Input: part model. Units: mm. Frame: model coordinates. A direction names the side the tool comes from. Round coordinates to 2 decimals unless told otherwise and drop trailing zeros. Loops run counter-clockwise (first coordinate to the right, second up) from the corner with the lowest first, then second, coordinate; pieces in that order, holes last.
(1) Cut plane D-D, the plane y = -6. Give the number of separate pieces and of enclosed holes in the cut face, and give its area (3 significant figures).
(2) Cut plane A-A, the plane z = -5. Output: boundary loops of the cut face in (x, y), and give its area (3 significant figures).
(3) Line query: line 1 (Y direction, x = 0, z = 14.7); line 2 (X direction, y = -4.5, z = 9); line 3 (Y direction, x = 6, z = 7.25). Output: solid intervals per line, ascending.
(4) Draft query along X for faces 1 (the face through (-0.22, 11.21, 13.82)), 2 (the face through (4.737, 0.052, -3.402)), 3 (the face through (0, -2, -6.9)), 4 (the face through (-1.5, -0.07, 1.63)). Return one class per face: released by +X, released by -X, zero draft, split by the parting line, or undercut.
(5) Cut plane C-C, the plane y = 0. Output: boundary loops of the cut face in (x, z).
(6) Access query for faces 5 (the face through (6.466, -2.681, 14.514)), 6 (the face through (-11.747, -4.917, 4.93)), 7 (the face through (3, 3.35, -3)), 8 (the face through (-4.737, -0.052, -3.402)). Directions: +Z, -Z, +X, -X, +Y, -Y. A direction counts if a zero-diameter tool reaches every point of the face in a straight line with its end or side. Return the directions, or none.
(7) First-contact query: pin 1 Ø4 at (x, y) = (8.25, -4.76) entering from +Z; pin 2 Ø8 at (x, z) = (10, 9.5) entering from +Y; pin 3 Ø5 at (x, y) = (0, 0) entering from +Z; pin 4 Ø10 at (x, z) = (-11.5, 12) entering from -Y. Flat tips, straight axial feed; report the tip coordinate or a pass-through.
from build123d import *

# Parameters (mm, degrees)
SKETCH_R        = 15
SKETCH_R_2      = 1.7
PAD_DEPTH       = 16
PAD001_DEPTH    = 6.9
SKETCH006_R     = 3.5
POCKET003_DEPTH = 6.9
SKETCH003_R     = 1.5
POCKET004_DEPTH = 17.3
SKETCH008_R     = 7
POCKET_DEPTH    = 2.5
SKETCH009_R     = 3.5
POCKET005_DEPTH = 10
CHAMFER_SIZE    = 1.5
CHAMFER001_SIZE = 1.7
CHAMFER002_SIZE = 1.7
CHAMFER003_SIZE = 1.7
CHAMFER004_SIZE = 0.5


with BuildPart() as part:
    # Sketch → Pad (new body)
    with BuildSketch(Plane.XY):
        Circle(SKETCH_R)
        with Locations((0, 9.526279)):
            Circle(SKETCH_R_2, mode=Mode.SUBTRACT)
        with Locations((-8.25, -4.76314)):
            Circle(SKETCH_R_2, mode=Mode.SUBTRACT)
        with Locations((8.25, -4.76314)):
            Circle(SKETCH_R_2, mode=Mode.SUBTRACT)
    extrude(amount=PAD_DEPTH)

    # Sketch004 → Pad001 (new body)
    with BuildSketch(Plane(origin=(0, 0, 0), x_dir=(1, 0, 0), z_dir=(0, 0, -1))):
        with BuildLine():
            Line((-3.35, 3.35), (3.35, 3.35))
            ThreePointArc((3.35, -3.35), (4.737615, 0), (3.35, 3.35))
            Line((3.35, -3.35), (-3.35, -3.35))
            ThreePointArc((-3.35, 3.35), (-4.737615, 0), (-3.35, -3.35))
        make_face()
    extrude(amount=PAD001_DEPTH)

    # Sketch006 → Pocket003 (cut)
    with BuildSketch(Plane(origin=(0, 0, -6.9), x_dir=(1, 0, 0), z_dir=(0, 0, -1))):
        with Locations((0, 6)):
            Circle(SKETCH006_R)
        with Locations((0, -6)):
            Circle(SKETCH006_R)
    extrude(amount=-POCKET003_DEPTH, mode=Mode.SUBTRACT)

    # Sketch003 → Pocket004 (cut)
    with BuildSketch(Plane(origin=(0, 0, -6.9), x_dir=(1, 0, 0), z_dir=(0, 0, -1))):
        Circle(SKETCH003_R)
    extrude(amount=-POCKET004_DEPTH, mode=Mode.SUBTRACT)

    # Sketch008 → Pocket (cut)
    with BuildSketch(Plane.XY.offset(16)):
        Circle(SKETCH008_R)
    extrude(amount=-POCKET_DEPTH, mode=Mode.SUBTRACT)

    # Sketch009 → Pocket005 (cut)
    with BuildSketch(Plane(origin=(0, 0, 0), x_dir=(1, 0, 0), z_dir=(0, 0, -1))):
        with Locations((8.25, 4.76314)):
            Circle(SKETCH009_R)
        with Locations((-8.25, 4.76314)):
            Circle(SKETCH009_R)
        with Locations((0, -9.526279)):
            Circle(SKETCH009_R)
    extrude(amount=-POCKET005_DEPTH, mode=Mode.SUBTRACT)

    # Chamfer
    chamfer_edges = [part.edges().sort_by_distance(p)[0] for p in [
        (-15, 0, 0),
    ]]
    chamfer(chamfer_edges, length=CHAMFER_SIZE)

    # Chamfer001
    chamfer001_edges = [part.edges().sort_by_distance(p)[0] for p in [
        (-9.95, -4.76314, 10),
    ]]
    chamfer(chamfer001_edges, length=CHAMFER001_SIZE)

    # Chamfer002
    chamfer002_edges = [part.edges().sort_by_distance(p)[0] for p in [
        (6.55, -4.76314, 10),
    ]]
    chamfer(chamfer002_edges, length=CHAMFER002_SIZE)

    # Chamfer003
    chamfer003_edges = [part.edges().sort_by_distance(p)[0] for p in [
        (-1.7, 9.526279, 10),
    ]]
    chamfer(chamfer003_edges, length=CHAMFER003_SIZE)

    # Chamfer004
    chamfer004_edges = [part.edges().sort_by_distance(p)[0] for p in [
        (-7, 0, 16),
    ]]
    chamfer(chamfer004_edges, length=CHAMFER004_SIZE)


solid = part.part
Reported:
1. separate pieces: 3
1. enclosed holes: 0
1. area: 253 mm2
2. outline: (-3.35, -3.35) - (-2.29, -3.35) arc R3.5 cw to (2.29, -3.35) - (3.35, -3.35) arc R4.74 ccw to (3.35, 3.35) - (2.29, 3.35) arc R3.5 cw to (-2.29, 3.35) - (-3.35, 3.35) arc R4.74 ccw to start; hole circle Ø3 at (0, 0)
2. area: 45.3 mm2
3. line 1: y = -15 to -7, 7 to 7.83, 11.23 to 15
3. line 2: x = -14.31 to -11.74, -4.76 to 4.76, 11.74 to 14.31
3. line 3: y = -13.75 to -7.44, -2.08 to 13.75
4. face 1: undercut
4. face 2: released by +X
4. face 3: zero draft
4. face 4: undercut
5. outline: (-15, 1.5) - (-13.5, 0) - (-4.74, 0) - (-4.74, -6.9) - (-1.5, -6.9) - (-1.5, 10.4) - (1.5, 10.4) - (1.5, -6.9) - (4.74, -6.9) - (4.74, 0) - (13.5, 0) - (15, 1.5) - (15, 16) - (7.5, 16) - (7, 15.5) - (7, 13.5) - (-7, 13.5) - (-7, 15.5) - (-7.5, 16) - (-15, 16) - close
6. face 5: +Z
6. face 6: -Z
6. face 7: -Z, +X, -X, +Y
6. face 8: -Z, -X
7. pin 1: stops at z = 16
7. pin 2: stops at y = 13.75
7. pin 3: stops at z = 13.5
7. pin 4: stops at y = -13.52
